Work out the finished part from the listing and answer in its coordinate system (mm). A direction names the side the tool comes from. Coordinates: 2 decimals unless noted, no trailing zeros. Order: outer loops, then holes, each group sorted by start corner. A loop starts at its lowest first (then second) coordinate and runs counter-clockwise, first axis right, second up. Notation, with made-up numbers: (-5, 24) - (35, 24) arc R18 ccw to (35, 52) - close; hole circle Ø5 at (86, 18.25). An arc over 180 degrees is marked (long way). Answer as a JSON object with one key per item and string values. Group by question number.
1) The mould has two halves that part along Y. Classify faces 1 (the face through (52, -62.045, 5)), 2 (the face through (21.703, -53.4, -0.4)), 3 (the face through (79.275, -45.496, -0.986)): released by +Y, released by -Y, zero draft, split by the parting line, or undercut.
2) A tool of negligible diameter and unlimited length cuts with its end or side. For faces 4 (the face through (52, -65, 0)), 5 (the face through (52, -43, 0)), 6 (the face through (79.975, -34.188, -0.986)), from which of +Z, -Z, +X, -X, +Y, -Y can it reach the whole face along a straight path? Write none if from no direction.
3) Each of these flat-tipped pins is pushed along its axis until it touches: P1, Ø5, axis at x = 62, z = 7, coming from the +Y side (3 decimals); P2, Ø1.7, axis at x = 75.12, y = -44.32, coming from the +Z side; P3, Ø1, axis at x = 70.5, z = 5.5, coming from the -Y side (3 decimals). Where does it stop, or does it pass through?
4) Section A-A (x = 53) is taken. Give the vertices of the cut face in (y, z).
5) Find the intervals of material crossed by line 1 along Z through (x, y) = (51.5, -41.5); line 2 along Y through (x, z) = (25.5, 1), in increasing order.
6) Section B-B (z = 3.25) is taken. Give the vertices of the cut face in (x, y), plus the area to 3 significant figures.
from build123d import *

# Parameters (mm, degrees)
ESQUISSE14_W       = 61.498402753
ESQUISSE14_H       = 40
ESQUISSE14_R       = 1.605618906
ESQUISSE14_R_2     = 1.680447067
ESQUISSE14_R_3     = 0.733091197
BOSS_EXTRU_1_DEPTH = 2
ESQUISSE15_W       = 61.498402753
ESQUISSE15_H       = 4
BOSS_EXTRU_2_DEPTH = 10


with BuildPart() as part:
    # Esquisse14 → Boss.-Extru.1 (new body)
    with BuildSketch(Plane.XY):
        with Locations((52.452549346, -48.865029397)):
            Rectangle(ESQUISSE14_W, ESQUISSE14_H)
        with Locations((78.443148937, -34.669848165)):
            Circle(ESQUISSE14_R, mode=Mode.SUBTRACT)
        with Locations((77.672120282, -46.000448366)):
            Circle(ESQUISSE14_R_2, mode=Mode.SUBTRACT)
        with Locations((29.018235202, -34.669848165)):
            Circle(ESQUISSE14_R_2, mode=Mode.SUBTRACT)
        with Locations((30.026503442, -52.148907634)):
            Circle(ESQUISSE14_R_2, mode=Mode.SUBTRACT)
        with Locations((75.118944162, -44.320001299)):
            Circle(ESQUISSE14_R_3, mode=Mode.SUBTRACT)
    extrude(amount=-BOSS_EXTRU_1_DEPTH)

    # Esquisse15 → Boss.-Extru.2 (add)
    with BuildSketch(Plane.XY):
        with Locations((52.452549346, -60.045029397)):
            Rectangle(ESQUISSE15_W, ESQUISSE15_H)
    extrude(amount=BOSS_EXTRU_2_DEPTH)


solid = part.part
Report:
{
 "1": {"face 1": "released by -Y", "face 2": "zero draft", "face 3": "undercut"},
 "2": {"face 4": "+Z, +X, -X, -Y", "face 5": "+Z, +X, -X, +Y", "face 6": "+Z, -Z"},
 "3": {"P1": "stops at y = -58.045", "P2": "stops at z = 0", "P3": "stops at y = -62.045"},
 "4": {"outline": "(-68.87, -2) - (-28.87, -2) - (-28.87, 0) - (-58.05, 0) - (-58.05, 10) - (-62.05, 10) - (-62.05, 0) - (-68.87, 0) - close"},
 "5": {"line 1": "z = -2 to 0", "line 2": "y = -62.05 to -58.05"},
 "6": {"outline": "(21.7, -62.05) - (83.2, -62.05) - (83.2, -58.05) - (21.7, -58.05) - close", "area": "246 mm²"}
}
